Build history of the part. All positions in model axes, mm. Face numbers are marked on the shaded views. A direction names the side the tool comes from. Give positions to 0.01 mm unless a question says otherwise; leave off trailing zeros. Loops run counter-clockwise (first coordinate to the right, second up) from the corner with the lowest first, then second, coordinate; pieces in that order, holes last. Notation, with made-up numbers: (55, 76) -> (76, 76) arc R25 ccw to (76, 98) -> close; hole circle Ø4 at (1, 80.5). An arc over 180 degrees is marked (long way). Answer as a JSON object with one key per item and string values. Group by question number.
Q1. Band-saw the part on D-D, the plane x = -10.25. Write the cut outline in (y, z).
Q2. Band-saw the part on A-A, the plane y = 15. Write the cut outline in (x, z), plus the area to 3 significant figures.
Q3. Drop flat-ended pins along their axis: pin 1 (1.5 mm diameter, centred on y = 3, z = 32, fed in from +X); pin 2 (2.5 mm diameter, centred on x = -1, y = 15.5, fed in from +Z); pin 3 (6 mm diameter, centred on x = -6, z = 6.5, fed in from -Y); pin 4 (1.9 mm diameter, centred on x = 0, y = 15, fed in from +Z). Give the stop position or say it passes through.
Q4. Tool access for the marked faces 1 and 2: list every direction of +Z, -Z, +X, -X, +Y, -Y with a clear straight run to the whole face (end or side of a thin tool).
Q5. Band-saw the part on C-C, the plane z = 11. Write the cut outline in (x, y), plus the area to 3 significant figures.
Q6. Wall check: probe 1 along Y at (x, z) = (0, 47); probe 2 along Y at (x, z) = (0, 52.75); probe 3 along X at (y, z) = (-15, 49). Give the ranges that are in metal, low to high. Write a range as from..to.
Q7. Band-saw the part on B-B, the plane y = 0. Write the cut outline in (x, z), plus the area to 3 significant figures.
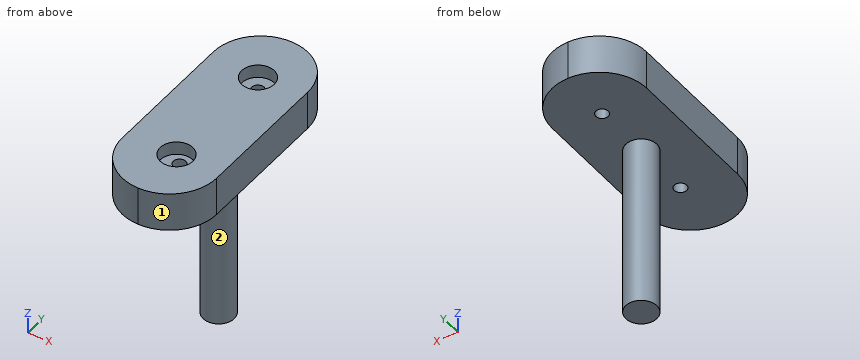
from build123d import *

# Parameters (mm, degrees)
SKETCH1_R             = 3.98
BOSS_EXTRUDE1_DEPTH   = 54.5
SKETCH3_W             = 24.26
SKETCH3_H             = 59.06
BOSS_EXTRUDE2_DEPTH   = 10
SKETCH4_R             = 1.6
CUT_EXTRUDE1_DEPTH    = 56.204619372
CROQUIS2_R            = 4.18
CORTAR_EXTRUIR2_DEPTH = 3.39
REDONDEO1_R           = 12.13


with BuildPart() as part:
    # Sketch1 → Boss-Extrude1 (new body)
    with BuildSketch(Plane.XY):
        Circle(SKETCH1_R)
    extrude(amount=BOSS_EXTRUDE1_DEPTH)

    # Sketch3 → Boss-Extrude2 (add)
    with BuildSketch(Plane.XY.offset(54.5)):
        with Locations((-0.57, -0.57)):
            Rectangle(SKETCH3_W, SKETCH3_H)
    extrude(amount=-BOSS_EXTRUDE2_DEPTH)

    # Sketch4 → Cut-Extrude1 (cut, through all)
    with BuildSketch(Plane(origin=(0, 0, 44.5), x_dir=(-1, 0, 0), z_dir=(0, 0, -1))):
        with Locations((0, 15)):
            Circle(SKETCH4_R)
        with Locations(Location((0, -15, 0), (0, 0, 180))):
            Circle(SKETCH4_R)
    extrude(amount=-CUT_EXTRUDE1_DEPTH, mode=Mode.SUBTRACT)

    # Croquis2 → Cortar-Extruir2 (cut)
    with BuildSketch(Plane.XY.offset(54.5)):
        with Locations((0, 15)):
            Circle(CROQUIS2_R)
        with Locations(Location((0, -16.14, 0), (0, 0, 180))):
            Circle(CROQUIS2_R)
    extrude(amount=-CORTAR_EXTRUIR2_DEPTH, mode=Mode.SUBTRACT)

    # Redondeo1
    redondeo1_edges = [part.edges().sort_by_distance(p)[0] for p in [
        (11.56, -30.1, 49.5),
        (-12.7, -30.1, 49.5),
        (-12.7, 28.96, 49.5),
        (11.56, 28.96, 49.5),
    ]]
    fillet(redondeo1_edges, radius=REDONDEO1_R - 0.0001)  # a hair under: the kernel refuses the full size


solid = part.part
Worked answers:
{
 "1": {"outline": "(-25.28, 44.5) -> (24.14, 44.5) -> (24.14, 54.5) -> (-25.28, 54.5) -> close"},
 "2": {"outline": "(-12.7, 44.5) -> (-1.6, 44.5) -> (-1.6, 51.11) -> (-4.18, 51.11) -> (-4.18, 54.5) -> (-12.7, 54.5) -> close; (1.6, 44.5) -> (11.56, 44.5) -> (11.56, 54.5) -> (4.18, 54.5) -> (4.18, 51.11) -> (1.6, 51.11) -> close", "area": "193 mm2"},
 "3": {"pin 1": "x = 3.28", "pin 2": "z = 51.11", "pin 3": "y = -2.62", "pin 4": "through"},
 "4": {"face 1": "+Z, -Z, +X, -Y", "face 2": "-Z"},
 "5": {"outline": "circle Ø7.96 at (0, 0)", "area": "49.8 mm2"},
 "6": {"probe 1": "-30.09..-16.6, -13.4..13.4, 16.6..28.95", "probe 2": "-30.09..-20.32, -11.96..10.82, 19.18..28.95", "probe 3": "-12.7..-1.6, 1.6..11.56"},
 "7": {"outline": "(-12.7, 44.5) -> (-3.98, 44.5) -> (-3.98, 0) -> (3.98, 0) -> (3.98, 44.5) -> (11.56, 44.5) -> (11.56, 54.5) -> (-12.7, 54.5) -> close", "area": "597 mm2"}
}
